Read the model definition and answer for the solid it produces. Units are mm, in the model's axes. Face numbers are marked on the shaded views. Round coordinates to 2 decimals unless told otherwise and drop trailing zeros. Write each loop counter-clockwise with the first axis right and the second up, starting at its lowest first coordinate (ties: lowest second). Pieces come first, ordered by that corner, then holes. Notation, with made-up numbers: (53, -3) -> (73, -3) arc R31 cw to (73, 36) -> close; hole circle Ø1 at (-23, -19). An arc over 180 degrees is marked (long way). Return JSON: item names as keys, results as strings. Group by question number.
(1) A cutting plane is placed at A-A on y = 76. Give the vertices of the cut face in (x, z), then the cut area to 4 significant figures.
(2) A cutting plane is placed at B-B on x = -2. Give the vertices of the cut face in (y, z), then the cut area to 3 significant figures.
(3) Given pin 1 (6 mm diameter, centred on x = -3, z = -4.5, fed in from -Y); pin 2 (7.5 mm diameter, centred on x = 0, y = 76, fed in from +Z), each flat-ended and moving along its own axis, determine where each tip first touches the part or whether it passes through.
(4) The mould has two halves that part along Y. Classify the marked faces 1, 2 and 3: released by +Y, released by -Y, zero draft, split by the parting line, or undercut.
(5) Straight lines are drawn through the part: line 1 (Y direction, x = 0, z = -1.25); line 2 (Y direction, x = -2.5, z = 0.75); line 3 (X direction, y = 72, z = -6.5). For each, find the intervals that lie inside material, in ascending order.
(6) A cutting plane is placed at C-C on z = 2. Give the vertices of the cut face in (x, y) (1 decimal), then the cut area to 3 significant figures.
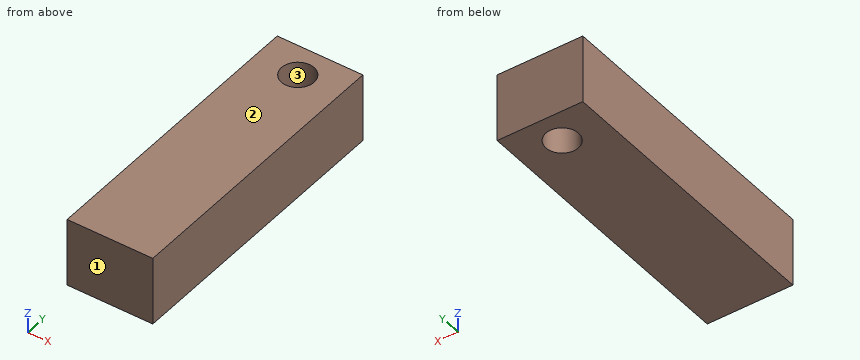
```python
from build123d import *

# Parameters (mm, degrees)
SKETCH1_W           = 25
SKETCH1_H           = 20
BOSS_EXTRUDE1_DEPTH = 85
SKETCH2_R           = 4.7625
CUT_EXTRUDE1_DEPTH  = 12


with BuildPart() as part:
    # Sketch1 → Boss-Extrude1 (new body)
    with BuildSketch(Plane(origin=(0, 0, 0), x_dir=(1, 0, 0), z_dir=(0, 1, 0))):
        Rectangle(SKETCH1_W, SKETCH1_H)
    extrude(amount=BOSS_EXTRUDE1_DEPTH)

    # Sketch2 → Cut-Extrude1 (cut, symmetric)
    with BuildSketch(Plane.XY):
        with Locations((0, 76)):
            Circle(SKETCH2_R)
    extrude(amount=CUT_EXTRUDE1_DEPTH, both=True, mode=Mode.SUBTRACT)


solid = part.part
```
Checks:
{
 "1": {"outline": "(-12.5, -10) -> (-4.76, -10) -> (-4.76, 10) -> (-12.5, 10) -> close; (4.76, -10) -> (12.5, -10) -> (12.5, 10) -> (4.76, 10) -> close", "area": "309.5 mm^2"},
 "2": {"outline": "(0, -10) -> (71.68, -10) -> (71.68, 10) -> (0, 10) -> close; (80.32, -10) -> (85, -10) -> (85, 10) -> (80.32, 10) -> close", "area": "1,530 mm^2"},
 "3": {"pin 1": "stops at y = 0", "pin 2": "passes through"},
 "4": {"face 1": "released by -Y", "face 2": "zero draft", "face 3": "undercut"},
 "5": {"line 1": "y = 0 to 71.24, 80.76 to 85", "line 2": "y = 0 to 71.95, 80.05 to 85", "line 3": "x = -12.5 to -2.58, 2.58 to 12.5"},
 "6": {"outline": "(-12.5, 0) -> (12.5, 0) -> (12.5, 85) -> (-12.5, 85) -> close; hole circle Ø9.5 at (0, 76)", "area": "2,050 mm^2"}
}
